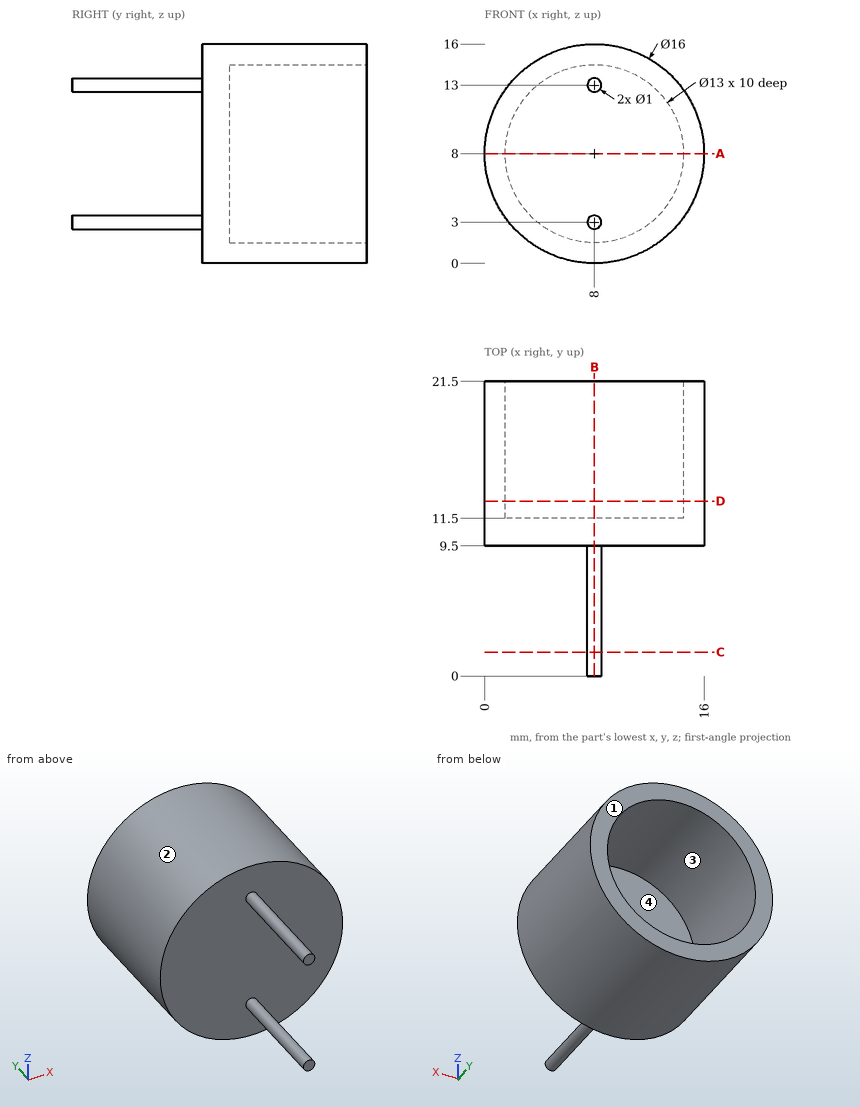
Check sheet for the drawn part. Datum: minimum x, y, z corner. Units: mm. Round coordinates to 2 decimals unless told otherwise and drop trailing zeros. Loops run counter-clockwise (first coordinate to the right, second up) from the corner with the lowest first, then second, coordinate; pieces in that order, holes last. Notation, with made-up numbers: (-24.75, 6.25) - (-14.75, 6.25) arc R26 ccw to (-14.75, 30.25) - close; hole circle Ø1 at (86, -36). An arc over 180 degrees is marked (long way). Answer as a JSON object with one key per item and string values. Group by question number.
Q1. Sectioned sample at B-B, the plane x = 8. Enter the section's corners in (y, z), plus the area to 3 significant figures.
Q2. Mould release check, pull along Z, two halves, no side actions. Record for the marked faces 1, 2, 3 and 4: released by +Z, released by -Z, zero draft, split by the parting line, or undercut.
Q3. Sectioned sample at A-A, the plane z = 8. Enter the section's corners in (x, y), plus the area to 3 significant figures.
Q4. Scan lines: line 1 along Z through (x, y) = (8, 16.5); line 2 along Y through (x, z) = (8.25, 6); line 3 along Y through (x, z) = (2.25, 13.5). Record each from-to range of solid material in increasing order. Write a range as [from, to].
Q5. Sectioned sample at D-D, the plane y = 12.75. Enter the section's corners in (x, z).
Q6. Sectioned sample at C-C, the plane y = 1.75. Enter the section's corners in (x, z).
Q7. Gauge pin test, flat ends, axial feed: P1, Ø1.5, axis at x = 7.5, z = 8, coming from the -Y side; P2, Ø6.5, axis at x = 7.5, z = 7.5, coming from the +Y side; P3, Ø1.5, axis at x = 5.5, y = 7.5, coming from the +Z side; P4, Ø1, axis at y = 18, z = 3, coming from the -X side. Record the tip position at first contact, or that the pin passes through.
Solution:
{
 "1": {"outline": "(0, 2.5) - (9.5, 2.5) - (9.5, 0) - (21.5, 0) - (21.5, 1.5) - (11.5, 1.5) - (11.5, 14.5) - (21.5, 14.5) - (21.5, 16) - (9.5, 16) - (9.5, 13.5) - (0, 13.5) - (0, 12.5) - (9.5, 12.5) - (9.5, 3.5) - (0, 3.5) - close", "area": "81.0 mm²"},
 "2": {"face 1": "zero draft", "face 2": "split by the parting line", "face 3": "undercut", "face 4": "undercut"},
 "3": {"outline": "(0, 9.5) - (16, 9.5) - (16, 21.5) - (14.5, 21.5) - (14.5, 11.5) - (1.5, 11.5) - (1.5, 21.5) - (0, 21.5) - close", "area": "62.0 mm²"},
 "4": {"line 1": "z = [0, 1.5], [14.5, 16]", "line 2": "y = [9.5, 11.5]", "line 3": "y = [9.5, 21.5]"},
 "5": {"outline": "circle Ø16 at (8, 8); hole circle Ø13 at (8, 8)"},
 "6": {"outline": "circle Ø1 at (8, 3); circle Ø1 at (8, 13)"},
 "7": {"P1": "stops at y = 9.5", "P2": "stops at y = 11.5", "P3": "passes through", "P4": "stops at x = 1.39"}
}
